from build123d import *

# Parameters (mm, degrees)
BOSS_EXTRUDE1_DEPTH = 9
FILLET3_R           = 1
SKETCH2_R           = 1.25
CUT_EXTRUDE1_DEPTH  = 3


with BuildPart() as part:
    # Sketch1 → Boss-Extrude1 (new body)
    with BuildSketch(Plane(origin=(0, 0, 0), x_dir=(1, 0, 0), z_dir=(0, 1, 0))):
        with BuildLine():
            Line((-15, 0), (15, 0))
            Line((15, 0), (28.906062556, 24.08600688))
            ThreePointArc((28.906062556, 24.08600688), (32.451975053, 24.443490384), (35.362311102, 26.500486732))
            Line((35.362311102, 26.500486732), (33.830222216, 27.786061952))
            ThreePointArc((33.830222216, 27.786061952), (25.016172377, 30.598176376), (33.265843673, 34.786061952))
            Line((33.265843673, 34.786061952), (34.572181143, 36.300486732))
            ThreePointArc((34.572181143, 36.300486732), (29.254107826, 37.9601469), (24.408479197, 35.211281884))
            Line((24.408479197, 35.211281884), (9, 5))
            Line((9, 5), (-9, 5))
            Line((-9, 5), (-24.408479197, 35.211281884))
            ThreePointArc((-24.408479197, 35.211281884), (-29.254107826, 37.9601469), (-34.572181143, 36.300486732))
            Line((-34.572181143, 36.300486732), (-33.265843673, 34.786061952))
            ThreePointArc((-33.265843673, 34.786061952), (-25.016172377, 30.598176376), (-33.830222216, 27.786061952))
            Line((-33.830222216, 27.786061952), (-35.362311102, 26.500486732))
            ThreePointArc((-35.362311102, 26.500486732), (-32.451975053, 24.443490384), (-28.906062556, 24.08600688))
            Line((-28.906062556, 24.08600688), (-15, 0))
        make_face()
        with BuildLine():
            Line((13.711166355, 9.835186109), (23.366165954, 28.765666577))
            ThreePointArc((23.366165954, 28.765666577), (24.748776454, 26.371322946), (26.950630684, 24.699099527))
            Line((26.950630684, 24.699099527), (17.309401077, 8))
            Line((17.309401077, 8), (13.711166355, 9.835186109))
        make_face(mode=Mode.SUBTRACT)
        with BuildLine():
            Line((-17.309401077, 8), (-13.711166355, 9.835186109))
            Line((-13.711166355, 9.835186109), (-23.366165954, 28.765666577))
            ThreePointArc((-23.366165954, 28.765666577), (-24.748776454, 26.371322946), (-26.950630684, 24.699099527))
            Line((-26.950630684, 24.699099527), (-17.309401077, 8))
        make_face(mode=Mode.SUBTRACT)
    extrude(amount=BOSS_EXTRUDE1_DEPTH)

    # Fillet3
    fillet3_edges = [part.edges().sort_by_distance(p)[0] for p in [
        (-33.265843673, 4.5, -34.786061952),
        (-34.572181143, 4.5, -36.300486732),
        (-33.830222216, 4.5, -27.786061952),
        (-35.362311102, 4.5, -26.500486732),
        (-17.309401077, 4.5, -8),
        (-13.711166355, 4.5, -9.835186109),
        (17.309401077, 4.5, -8),
        (13.711166355, 4.5, -9.835186109),
        (33.265843673, 4.5, -34.786061952),
        (34.572181143, 4.5, -36.300486732),
        (33.830222216, 4.5, -27.786061952),
        (35.362311102, 4.5, -26.500486732),
        (-9, 4.5, -5),
        (9, 4.5, -5),
    ]]
    fillet(fillet3_edges, radius=FILLET3_R - 0.0001)  # a hair under: the kernel refuses the full size

    # Sketch2 → Cut-Extrude1 (cut)
    with BuildSketch(Plane.XY):
        with Locations((-12, 4.5)):
            Circle(SKETCH2_R)
        with Locations((12, 4.5)):
            Circle(SKETCH2_R)
    extrude(amount=-CUT_EXTRUDE1_DEPTH, mode=Mode.SUBTRACT)


solid = part.part
Part model, mm, in its own coordinate system. A direction names the side the tool comes from. Coordinates: 2 decimals unless noted, no trailing zeros. Loops run counter-clockwise (first coordinate to the right, second up) from the corner with the lowest first, then second, coordinate; pieces in that order, holes last. Notation, with made-up numbers: (48, -9) -> (91, -9) arc R16 cw to (91, 22) -> close; hole circle Ø6 at (11.25, 53.25). An arc over 180 degrees is marked (long way). Use a Markdown table: item, result. Add a question column.
Item 1: Probe probe 1 along Z at (x, y) = (30, 6); probe 2 along X at (y, z) = (5.75, -18); probe 3 along Y at (x, z) = (12, -1). List the from-to ranges inside material, lowest first.
Item 2: Band-saw the part on C-C on z = -11.5. Write the cut outline in (x, y).
Item 3: Band-saw the part on A-A on x = -30. Write the cut outline in (y, z), plus the area to 3 significant figures.
Item 4: Band-saw the part on B-B on z = -30.5. Write the cut outline in (x, y).
Item 5: Band-saw the part on D-D on x = 7.5. Write the cut outline in (y, z).
Item 6: Which spindle directions (+Z, -Z, +X, -X, +Y, -Y) get a long thin tool onto all of the face, cutting with end or side? Do faces 1 (the flat face through (0, 4, 0)), 2 (the cylindrical face through (11.73, 3.28, -1.48)), 3 (the cylindrical face through (33.254, 4.563, -35.144)), 4 (the flat face through (16.95, 4.44, -20.59)). Say none if no direction does.
Item 7: Pull direction Z, two halves, no side cores. Call faces 5 (the cylindrical face through (33.9, 4.56, -27.43)), 6 (the flat face through (-12, 5, -3)), 7 (the cylindrical face through (-28.6, 4.44, -37.86)): +Z half, -Z half, draft (parallel to the pull), parting line (faces both ways), or undercut.
Item 8: Flat gauge pins, fed straight in: P1, Ø1.5, axis at x = 13, y = 8, coming from the -Z side; P2, Ø2, axis at x = 2.5, y = 6.5, coming from the -Z side; P3, Ø3, axis at y = 5, z = -12, coming from the +X side. Where does each tip first touch, or does it go through?
Geometry says:
| question | item | result |
|---|---|---|
| 1 | probe 1 | -38 to -36, -26 to -24 |
| 1 | probe 2 | -25.39 to -23.08, -17.88 to -15.63, 15.63 to 17.88, 23.08 to 25.39 |
| 1 | probe 3 | 0 to 3.25, 5.75 to 9 |
| 2 | outline | (-21.64, 0) -> (-19.33, 0) -> (-19.33, 9) -> (-21.64, 9) -> close; (-14.56, 0) -> (-12.32, 0) -> (-12.32, 9) -> (-14.56, 9) -> close; (12.32, 0) -> (14.56, 0) -> (14.56, 9) -> (12.32, 9) -> close; (19.33, 0) -> (21.64, 0) -> (21.64, 9) -> (19.33, 9) -> close |
| 3 | outline | (0, -38) -> (9, -38) -> (9, -36) -> (0, -36) -> close; (0, -26) -> (9, -26) -> (9, -24) -> (0, -24) -> close |
| 3 | area | 36.0 mm² |
| 4 | outline | (-25.03, 0) -> (-22.01, 0) -> (-22.01, 9) -> (-25.03, 9) -> close; (22.01, 0) -> (25.03, 0) -> (25.03, 9) -> (22.01, 9) -> close |
| 5 | outline | (0, -5) -> (9, -5) -> (9, 0) -> (0, 0) -> close |
| 6 | face 1 | +Z, +X, -X, +Y, -Y |
| 6 | face 2 | +Z |
| 6 | face 3 | +Y, -Y |
| 6 | face 4 | -Z, +Y, -Y |
| 7 | face 5 | undercut |
| 7 | face 6 | +Z half |
| 7 | face 7 | -Z half |
| 8 | P1 | z = -14.31 |
| 8 | P2 | z = -5 |
| 8 | P3 | x = 22.79 |
